Work out the finished part from the listing and answer in its coordinate system (mm). A direction names the side the tool comes from. Give positions to 0.01 mm unless a question says otherwise; leave off trailing zeros. Loops run counter-clockwise (first coordinate to the right, second up) from the corner with the lowest first, then second, coordinate; pieces in that order, holes last. Notation, with made-up numbers: M 34.5,9 L 50.5,9 A10 cw 50.5,22 Z; hole C 42.25,9 d3. An arc over 180 degrees is marked long. Write item = value, one per line. Start each with the question number.
1. The mould has two halves that part along Z. Classify faces 3 (the face through (48, 1.957, -46)), 4 (the face through (9.177, -33, 18)), 5 (the face through (83, -35, -47.696)): released by +Z, released by -Z, zero draft, split by the parting line, or undercut.
2. For faces 1 (the face through (83, -35, 82.804)), 2 (the face through (81, -33, 80.304)), determine the directions among +Z, -Z, +X, -X, +Y, -Y from which every point of the face is accessible in a straight line to the end or side of a thin tool.
3. Section A-A on y = -7.5 is taken. Determine the outline of the cut face in (x, z), plus the area to 3 significant figures.
4. A flat-ended cylindrical pin translates along its axis: pin 1 Ø4 at (x, z) = (86.5, 9.5) entering from +Y. Find the tip coordinate at first contact, or state that the pin passes through.
5. Section C-C on x = 113 is taken. Determine the outline of the cut face in (y, z), plus the area to 3 significant figures.
6. Section B-B on z = -13.5 is taken. Determine the outline of the cut face in (x, y), plus the area to 3 significant figures.
7. Consider L1, parallel to X at y = -28, z = 31; L2, parallel to Z at x = 13.5, y = -17; L3, parallel to Y at x = 24, z = -11. Determine where each line is inside the solid, lowest interval first. Write a range as [from, to].
```python
from build123d import *

# Parameters (mm, degrees)
SKETCH1_W           = 150.5
SKETCH1_H           = 130.5
SKETCH1_W_2         = 145.5
SKETCH1_H_2         = 125.5
BOSS_EXTRUDE1_DEPTH = 71.58
SKETCH3_W           = 150.5
SKETCH3_H           = 130.5
BOSS_EXTRUDE2_DEPTH = 2.5


with BuildPart() as part:
    # Sketch1 → Boss-Extrude1 (new body)
    with BuildSketch(Plane(origin=(0, 1.956589097, 0), x_dir=(1, 0, 0), z_dir=(0, 1, 0))):
        with Locations((81.927421255, -17.554481305)):
            Rectangle(SKETCH1_W, SKETCH1_H)
        with Locations((81.927421255, -17.554481305)):
            Rectangle(SKETCH1_W_2, SKETCH1_H_2, mode=Mode.SUBTRACT)
    extrude(amount=-BOSS_EXTRUDE1_DEPTH)

    # Sketch3 → Boss-Extrude2 (add)
    with BuildSketch(Plane(origin=(0, -69.623410903, 0), x_dir=(-1, 0, 0), z_dir=(0, -1, 0))):
        with Locations((-81.927421255, -17.554481305)):
            Rectangle(SKETCH3_W, SKETCH3_H)
    extrude(amount=BOSS_EXTRUDE2_DEPTH)


solid = part.part
```
Verdict:
q1.face_3 = zero draft
q1.face_4 = undercut
q1.face_5 = released by -Z
q2.face_1 = +Z, +X, -X, +Y, -Y
q2.face_2 = +Y
q3.outline = M 6.68,-47.7 L 157.18,-47.7 L 157.18,82.8 L 6.68,82.8 Z; hole M 9.18,-45.2 L 154.68,-45.2 L 154.68,80.3 L 9.18,80.3 Z
q3.area = 1,380 mm2
q4.pin_1 = -69.62
q5.outline = M -72.12,-47.7 L 1.96,-47.7 L 1.96,-45.2 L -69.62,-45.2 L -69.62,80.3 L 1.96,80.3 L 1.96,82.8 L -72.12,82.8 Z
q5.area = 684 mm2
q6.outline = M 6.68,-72.12 L 157.18,-72.12 L 157.18,1.96 L 154.68,1.96 L 154.68,-69.62 L 9.18,-69.62 L 9.18,1.96 L 6.68,1.96 Z
q6.area = 734 mm2
q7.L1 = [6.68, 9.18], [154.68, 157.18]
q7.L2 = [-47.7, -45.2], [80.3, 82.8]
q7.L3 = [-72.12, -69.62]
